Work out the finished part from the listing and answer in its coordinate system (mm). A direction names the side the tool comes from. Coordinates: 2 decimals unless noted, no trailing zeros. Use a Markdown table: item, result.
from build123d import *

# Parameters (mm, degrees)
F1_DEPTH = 10
F2_R     = 10
F3_R     = 120
F4_T     = -5
F5_R     = 5
F7_DEPTH = 2
F8_R     = 2
F9_R     = 2


with BuildPart() as f1:
    # F0 (on Top) → F1 (new body)
    with BuildSketch(Plane.XY):
        with BuildLine():
            Line((0, 85), (-28, 58.6600375042))
            ThreePointArc((-28, 58.6600375042), (0, -65), (28, 58.6600375042))
            Line((28, 58.6600375042), (0, 85))
        make_face()
    extrude(amount=F1_DEPTH)

    # F2
    f2_edges = [f1.edges().sort_by_distance(p)[0] for p in [
        (0, 85, 5),
    ]]
    fillet(f2_edges, radius=F2_R)

    # F3
    f3_edges = [f1.edges().sort_by_distance(p)[0] for p in [
        (-28, 58.660038, 5),
        (28, 58.660038, 5),
    ]]
    fillet(f3_edges, radius=F3_R)

    # F4
    f4_openings = [f1.faces().sort_by_distance(p)[0] for p in [
        (0, 2.490227, 0),
    ]]
    offset(amount=F4_T, openings=f4_openings)

    # F5
    f5_edges = [f1.edges().sort_by_distance(p)[0] for p in [
        (0, -65, 10),
        (12.376367, 73.357391, 10),
        (26.230576, 61.013655, 10),
        (0, 81.270685, 10),
        (-12.376367, 73.357391, 10),
        (-26.230576, 61.013655, 10),
    ]]
    fillet(f5_edges, radius=F5_R)

    # F6 (on face) → F7 (cut)
    with BuildSketch(Plane.XY.offset(10)):
        with BuildLine():
            Line((24.5830141958, -28.6241205137), (24.5830141958, 28.6241205137))
            ThreePointArc((24.5830141958, 28.6241205137), (4.5140931022, 24.9911712124), (-13.0076974051, 14.5534141782))
            Line((-13.0076974051, 14.5534141782), (-13.0076974051, 28))
            Line((-13.0076974051, 28), (-19.0571866046, 28))
            Line((-19.0571866046, 28), (-19.0571866046, -28))
            Line((-19.0571866046, -28), (-13.0076974051, -28))
            Line((-13.0076974051, -28), (-13.0076974051, -14.5534141782))
            ThreePointArc((-13.0076974051, -14.5534141782), (-7.6208581173, -18.7073881119), (-1.7793276831, -22.1930816072))
            ThreePointArc((-1.7793276831, -22.1930816072), (1.5769915618, -43.1576186172), (16.4944786534, -28.0498302354))
            ThreePointArc((16.4944786534, -28.0498302354), (20.5285655112, -28.4803674588), (24.5830141958, -28.6241205137))
        make_face()
        with BuildLine():
            ThreePointArc((11.9329452437, -27.2089956114), (2.7197472284, -39.5920744788), (2.4211464703, -24.1604673852))
            ThreePointArc((2.4211464703, -24.1604673852), (7.1104323918, -25.8925740471), (11.9329452437, -27.2089956114))
        make_face(mode=Mode.SUBTRACT)
    extrude(amount=-F7_DEPTH, mode=Mode.SUBTRACT)

    # F8
    f8_edges = [f1.edges().sort_by_distance(p)[0] for p in [
        (-13.007697, 28, 9),
        (-19.057187, 28, 9),
        (-13.007697, 14.553414, 9),
        (24.583014, 28.624121, 9),
        (24.583014, -28.624121, 9),
        (16.494479, -28.04983, 9),
        (-1.779328, -22.193082, 9),
        (2.421146, -24.160467, 9),
        (11.932945, -27.208996, 9),
        (-13.007697, -14.553414, 9),
        (-13.007697, -28, 9),
        (-19.057187, -28, 9),
    ]]
    fillet(f8_edges, radius=F8_R)

    # F9
    f9_edges = [f1.edges().sort_by_distance(p)[0] for p in [
        (0, -65, 0),
        (-26.230576, 61.013655, 0),
        (26.230576, 61.013655, 0),
        (-12.376367, 73.357391, 0),
        (12.376367, 73.357391, 0),
        (0, 81.270685, 0),
        (8.950439, 69.715549, 0),
        (23.151719, 57.074031, 0),
        (0, -60, 0),
        (-23.151719, 57.074031, 0),
        (-8.950439, 69.715549, 0),
        (0, 76.270685, 0),
    ]]
    fillet(f9_edges, radius=F9_R)


solid = f1.part
(1) Which of the six approach directions +Z, -Z, +X, -X, +Y, -Y give full straight-line access (tool end or side, diameter ignored) to faces 1 (the cylindrical face through (-26.11, 61.11, 3.52)), 2 (the flat face through (9.03, 69.64, 3.48)), 3 (the cylindrical face through (5.705, 25.422, 9.014))?
Conclusion:
| item | result |
|---|---|
| face 1 | +Z, -Z, -X, +Y |
| face 2 | -Z |
| face 3 | +Z |
(2) Straight lines are drawn through the part: L1, parallel to X at y = 0, z = 4.05; L2, parallel to X at y = -34, z = 8.5; L3, parallel to Z at x = 23, y = 42.5. For each, find the intervals that lie inside material, in ascending order.
Conclusion:
| item | result |
|---|---|
| L1 | -65 to -60, 60 to 65 |
| L2 | -53.71 to -6.49, -2.65 to 13.07, 16.91 to 53.71 |
| L3 | 5 to 10 |
(3) Given P1, Ø2, axis at y = 4.5, z = 9.5, coming from the -X side; P2, Ø4, axis at x = 23.5, z = 1, coming from the +Y side; P3, Ø2, axis at x = -16.5, z = 8.5, coming from the -Y side, each flat-ended and moving along its own axis, determine where each tip first touches the part or whether it passes through.
Conclusion:
| item | result |
|---|---|
| P1 | x = -63.41 |
| P2 | y = 64.78 |
| P3 | y = -62.23 |
(4) Determine the mould class of faces 4 (the flat face through (5, -32, 10)), 5 (the flat face through (-1, 9, 5)), 6 (the cylindrical face through (-0.11, 81.27, 3.52)) for opening direction Y: pulls with the +Y half, pulls with the -Y half, needs draft (parallel to the pull), parting line crosses it, or undercut.
Conclusion:
| item | result |
|---|---|
| face 4 | needs draft |
| face 5 | undercut |
| face 6 | pulls with the +Y half |
